from build123d import *

# Parameters (mm, degrees)
SKETCH_1_W               = 366
SKETCH_1_H               = 566
EXTRUDE_1_DEPTH          = 3
SKETCH_5_R               = 2.25
CUT_EXTRUDE_2_DEPTH      = 4
SKETCH_8_R               = 4
CUT_EXTRUDE_5_DEPTH      = 4
CUT_EXTRUDE_5_DEPTH_BACK = 10
SKETCH_10_R              = 2.25
CUT_EXTRUDE_6_DEPTH      = 4
SKETCH_11_R              = 4
CUT_EXTRUDE_7_DEPTH      = 4


with BuildPart() as part:
    # Эскиз1 → Бобышка-Вытянуть1 (new body)
    with BuildSketch(Plane.XY):
        with Locations((183, 283)):
            Rectangle(SKETCH_1_W, SKETCH_1_H)
    extrude(amount=EXTRUDE_1_DEPTH)

    # Эскиз5 → Вырез-Вытянуть2 (cut, through all)
    with BuildSketch(Plane(origin=(0, 0, 0), x_dir=(-1, 0, 0), z_dir=(0, 0, -1))):
        with Locations((-353, 553)):
            Circle(SKETCH_5_R)
        with Locations((-13, 553)):
            Circle(SKETCH_5_R)
        with Locations((-243, 553)):
            Circle(SKETCH_5_R)
        with Locations((-123, 553)):
            Circle(SKETCH_5_R)
        with Locations((-353, 418)):
            Circle(SKETCH_5_R)
        with Locations((-353, 283)):
            Circle(SKETCH_5_R)
        with Locations((-353, 148)):
            Circle(SKETCH_5_R)
        with Locations((-353, 13)):
            Circle(SKETCH_5_R)
        with Locations((-123, 13)):
            Circle(SKETCH_5_R)
        with Locations((-243, 13)):
            Circle(SKETCH_5_R)
        with Locations((-13, 418)):
            Circle(SKETCH_5_R)
        with Locations((-13, 283)):
            Circle(SKETCH_5_R)
        with Locations((-13, 148)):
            Circle(SKETCH_5_R)
        with Locations((-13, 13)):
            Circle(SKETCH_5_R)
    extrude(amount=-CUT_EXTRUDE_2_DEPTH, mode=Mode.SUBTRACT)

    # Эскиз8 → Вырез-Вытянуть5 (cut, two sides)
    with BuildSketch(Plane.XY) as cut_extrude_5_sk:
        with Locations((305, 148.5)):
            Circle(SKETCH_8_R)
        with Locations((313.485281374, 162.514718626)):
            Circle(SKETCH_8_R)
        with Locations((305, 171)):
            Circle(SKETCH_8_R)
        with Locations((293.75, 151.514428415)):
            Circle(SKETCH_8_R)
        with Locations((285.514428415, 159.75)):
            Circle(SKETCH_8_R)
        with Locations((282.5, 171)):
            Circle(SKETCH_8_R)
        with Locations((285.514428415, 182.25)):
            Circle(SKETCH_8_R)
        with Locations((293.75, 190.485571585)):
            Circle(SKETCH_8_R)
        with Locations((305, 193.5)):
            Circle(SKETCH_8_R)
        with Locations((316.25, 190.485571585)):
            Circle(SKETCH_8_R)
        with Locations((324.485571585, 182.25)):
            Circle(SKETCH_8_R)
        with Locations((327.5, 171)):
            Circle(SKETCH_8_R)
        with Locations((324.485571585, 159.75)):
            Circle(SKETCH_8_R)
        with Locations((316.25, 151.514428415)):
            Circle(SKETCH_8_R)
        with Locations((301.894171459, 159.408890085)):
            Circle(SKETCH_8_R)
        with Locations((293.408890085, 167.894171459)):
            Circle(SKETCH_8_R)
        with Locations((296.514718626, 179.485281374)):
            Circle(SKETCH_8_R)
        with Locations((308.105828541, 182.591109915)):
            Circle(SKETCH_8_R)
        with Locations((316.591109915, 174.105828541)):
            Circle(SKETCH_8_R)
        with Locations((272.5, 73)):
            Circle(SKETCH_8_R)
        with Locations((272.5, 50.5)):
            Circle(SKETCH_8_R)
        with Locations((280.985281374, 64.514718626)):
            Circle(SKETCH_8_R)
        with Locations((261.25, 53.514428415)):
            Circle(SKETCH_8_R)
        with Locations((253.014428415, 61.75)):
            Circle(SKETCH_8_R)
        with Locations((250, 73)):
            Circle(SKETCH_8_R)
        with Locations((253.014428415, 84.25)):
            Circle(SKETCH_8_R)
        with Locations((261.25, 92.485571585)):
            Circle(SKETCH_8_R)
        with Locations((272.5, 95.5)):
            Circle(SKETCH_8_R)
        with Locations((283.75, 92.485571585)):
            Circle(SKETCH_8_R)
        with Locations((291.985571585, 84.25)):
            Circle(SKETCH_8_R)
        with Locations((295, 73)):
            Circle(SKETCH_8_R)
        with Locations((291.985571585, 61.75)):
            Circle(SKETCH_8_R)
        with Locations((283.75, 53.514428415)):
            Circle(SKETCH_8_R)
        with Locations((269.394171459, 61.408890085)):
            Circle(SKETCH_8_R)
        with Locations((260.908890085, 69.894171459)):
            Circle(SKETCH_8_R)
        with Locations((264.014718626, 81.485281374)):
            Circle(SKETCH_8_R)
        with Locations((275.605828541, 84.591109915)):
            Circle(SKETCH_8_R)
        with Locations((284.091109915, 76.105828541)):
            Circle(SKETCH_8_R)
    extrude(amount=CUT_EXTRUDE_5_DEPTH, mode=Mode.SUBTRACT)
    extrude(cut_extrude_5_sk.sketch, amount=-CUT_EXTRUDE_5_DEPTH_BACK, mode=Mode.SUBTRACT)

    # Эскиз10 → Вырез-Вытянуть6 (cut, through all)
    with BuildSketch(Plane.XY.offset(3)):
        with Locations((183, 470)):
            Circle(SKETCH_10_R)
        with Locations((183, 333)):
            Circle(SKETCH_10_R)
    extrude(amount=-CUT_EXTRUDE_6_DEPTH, mode=Mode.SUBTRACT)

    # Эскиз11 → Вырез-Вытянуть7 (cut, through all)
    with BuildSketch(Plane(origin=(0, 0, 0), x_dir=(-1, 0, 0), z_dir=(0, 0, -1))):
        with Locations((-63, 268)):
            Circle(SKETCH_11_R)
        with Locations((-63, 245.5)):
            Circle(SKETCH_11_R)
        with Locations((-71.485281374, 259.514718626)):
            Circle(SKETCH_11_R)
        with Locations((-74.25, 248.514428415)):
            Circle(SKETCH_11_R)
        with Locations((-82.485571585, 256.75)):
            Circle(SKETCH_11_R)
        with Locations((-85.5, 268)):
            Circle(SKETCH_11_R)
        with Locations((-82.485571585, 279.25)):
            Circle(SKETCH_11_R)
        with Locations((-74.25, 287.485571585)):
            Circle(SKETCH_11_R)
        with Locations((-63, 290.5)):
            Circle(SKETCH_11_R)
        with Locations((-51.75, 287.485571585)):
            Circle(SKETCH_11_R)
        with Locations((-43.514428415, 279.25)):
            Circle(SKETCH_11_R)
        with Locations((-40.5, 268)):
            Circle(SKETCH_11_R)
        with Locations((-43.514428415, 256.75)):
            Circle(SKETCH_11_R)
        with Locations((-51.75, 248.514428415)):
            Circle(SKETCH_11_R)
        with Locations((-74.591109915, 271.105828541)):
            Circle(SKETCH_11_R)
        with Locations((-66.105828541, 279.591109915)):
            Circle(SKETCH_11_R)
        with Locations((-54.514718626, 276.485281374)):
            Circle(SKETCH_11_R)
        with Locations((-51.408890085, 264.894171459)):
            Circle(SKETCH_11_R)
        with Locations((-59.894171459, 256.408890085)):
            Circle(SKETCH_11_R)
    extrude(amount=-CUT_EXTRUDE_7_DEPTH, mode=Mode.SUBTRACT)


solid = part.part
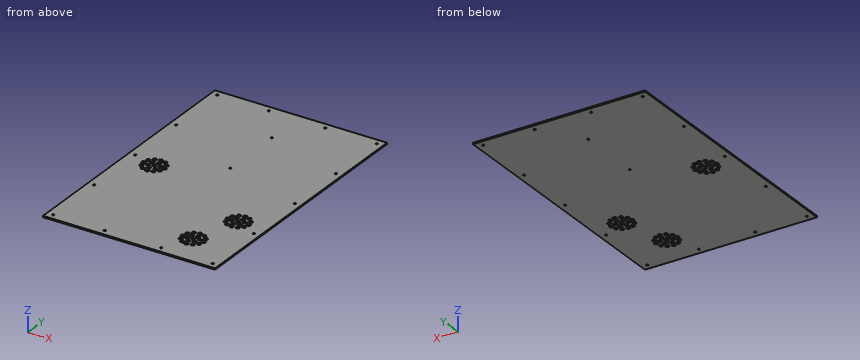
Work out the finished part from the listing and answer in its coordinate system (mm). Give positions to 0.01 mm unless a question says otherwise; leave off trailing zeros. Use a Markdown table: item, result. Add a question column.
1) Consider line 1 along X through (y, z) = (553, 1.85); line 2 along Y through (x, z) = (13, 2); line 3 along Y through (x, z) = (81, 0.65). Determine where each line is inside the solid, lowest interval first.
2) This flat-tipped pin is pushed along its axis until it touches: P1, Ø10.5, axis at x = 324.49, y = 182.25, coming from the -Z side. Where does it stop, or does it pass through?
3) The part is cut by section A-A, the plane z = 1.1. Count the separate pieces of the cut face and the enclosed holes in it, plus the area to 3 significant figures.
Reported:
| question | item | result |
|---|---|---|
| 1 | line 1 | x = 0 to 10.75, 15.25 to 120.75, 125.25 to 240.75, 245.25 to 350.75, 355.25 to 366 |
| 1 | line 2 | y = 0 to 10.75, 15.25 to 145.75, 150.25 to 280.75, 285.25 to 415.75, 420.25 to 550.75, 555.25 to 566 |
| 1 | line 3 | y = 0 to 253.04, 260.46 to 275.54, 282.96 to 566 |
| 2 | P1 | stops at z = 0 |
| 3 | separate pieces | 1 |
| 3 | enclosed holes | 73 |
| 3 | area | 204,000 mm^2 |
